Part print with two shaded views. Sizes in mm from the minimum x, y, z corner. Give positions to 0.01 mm unless a question says otherwise; leave off trailing zeros. Order: outer loops, then holes, each group sorted by start corner. A loop starts at its lowest first (then second) coordinate and runs counter-clockwise, first axis right, second up. Notation, with made-up numbers: (60, -40) -> (94, -40) arc R19 cw to (94, -34) -> close; hole circle Ø11 at (-27.75, 19). An arc over 180 degrees is marked (long way). Write item = value, one per line. Start each with the question number.
Item 1: Flat gauge pins, fed straight in: P1, Ø1.5, axis at x = 42.34, y = 2.39, coming from the -Z side; P2, Ø1.5, axis at x = 20, y = 4.5, coming from the -Z side; P3, Ø1, axis at y = 3, z = 2, coming from the +X side. Where does each tip first touch, or does it go through?
Item 2: Band-saw the part on B-B on z = 0.85. Count the separate pieces of the cut face and the enclosed holes in it, plus the area to 3 significant figures.
Item 3: Band-saw the part on C-C on y = 0.5. Write the cut outline in (x, z) (1 decimal).
Item 4: Drill centre lines: line 1 along X through (y, z) = (2.3, 2) (1 decimal); line 2 along X through (y, z) = (1.5, 2.3) (1 decimal); line 3 along X through (y, z) = (0.8, 1.25) (1 decimal). Where is each one in solid material? Low to high.
Item 5: Band-saw the part on A-A on y = 3.2. Write the cut outline in (x, z) (1 decimal).
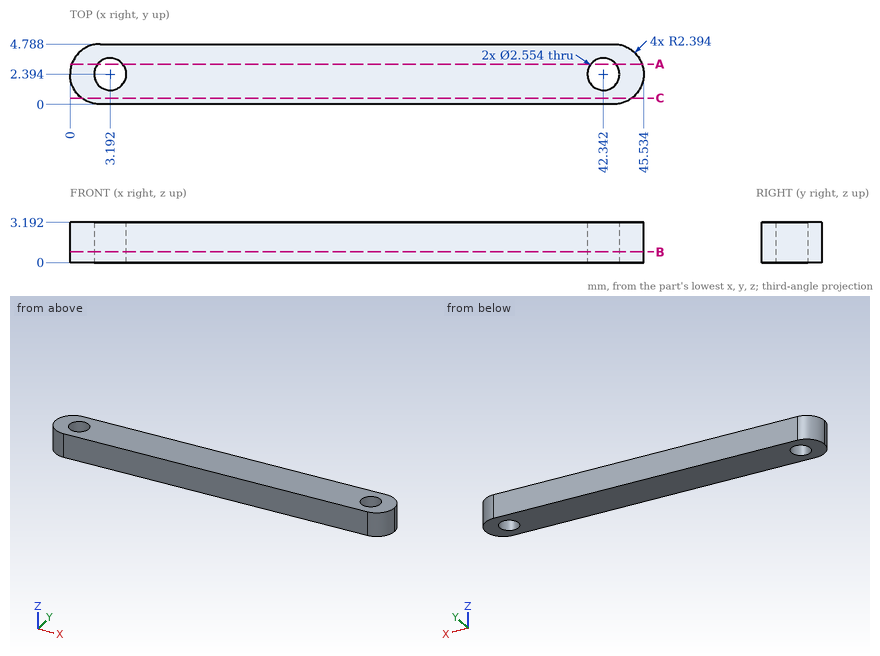
Values found:
q1.P1 = through
q1.P2 = 0
q1.P3 = 45.53
q2.separate_pieces = 1
q2.enclosed_holes = 2
q2.area = 203 mm^2
q3.outline = (0.9, 0) -> (44.6, 0) -> (44.6, 3.2) -> (0.9, 3.2) -> close
q4.line_1 = 0 to 1.9, 4.5 to 41.1, 43.6 to 45.5
q4.line_2 = 0.2 to 2.3, 4.1 to 41.4, 43.3 to 45.4
q4.line_3 = 0.6 to 44.9
q5.outline = (0.1, 0) -> (2.2, 0) -> (2.2, 3.2) -> (0.1, 3.2) -> close; (4.2, 0) -> (41.4, 0) -> (41.4, 3.2) -> (4.2, 3.2) -> close; (43.3, 0) -> (45.4, 0) -> (45.4, 3.2) -> (43.3, 3.2) -> close
